The listing builds one solid part. Answer for the finished solid, in the listing's coordinates (mm). Face numbers are marked on the shaded views. A direction names the side the tool comes from. Coordinates: 2 decimals unless noted, no trailing zeros. Write each loop counter-clockwise with the first axis right and the second up, starting at its lowest first coordinate (ties: lowest second). Pieces come first, ordered by that corner, then holes. Notation, with made-up numbers: M -33.5,-2.75 L 18.5,-2.75 A24 cw 18.5,13.25 Z; hole C 34.25,53 d3. An arc over 180 degrees is marked long. Answer as a JSON object with one key per item and string values. Group by question number.
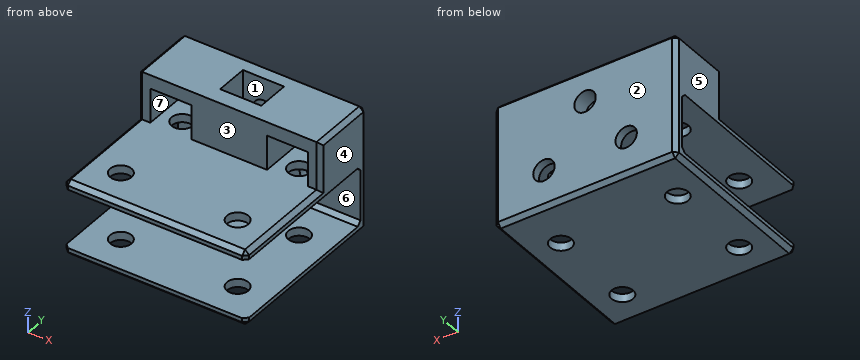
from build123d import *

# Parameters (mm, degrees)
SKETCH1_W           = 44.4
SKETCH1_H           = 40
SKETCH1_R           = 2.6
BOSS_EXTRUDE1_DEPTH = 2
SKETCH2_W           = 44.4
SKETCH2_H           = 18.3
BOSS_EXTRUDE2_DEPTH = 2
LPATTERN1_COUNT     = 2
LPATTERN1_PITCH     = 16.3
SKETCH3_R           = 2.6
CUT_EXTRUDE1_DEPTH  = 64.253853638
BOSS_EXTRUDE3_START = -22.2
SKETCH6_W           = 11.69
SKETCH6_H           = 16
BOSS_EXTRUDE3_DEPTH = 44.4
FILLET4_SIZE        = 1
SKETCH12_W          = 10
SKETCH12_H          = 8.384441544
CUT_EXTRUDE7_DEPTH  = 11
SKETCH11_R          = 2.6
CUT_EXTRUDE8_DEPTH  = 10
CUT_EXTRUDE9_REACH  = 70.079
SKETCH13_W          = 10
SKETCH13_H          = 8


with BuildPart() as part:
    # Sketch1 → Boss-Extrude1 (new body)
    with BuildSketch(Plane.XY):
        with Locations((22.2, 20)):
            Rectangle(SKETCH1_W, SKETCH1_H)
        with Locations((8, 8.476902454)):
            Circle(SKETCH1_R, mode=Mode.SUBTRACT)
        with Locations((8, 29.976902454)):
            Circle(SKETCH1_R, mode=Mode.SUBTRACT)
        with Locations((36.4, 29.976902454)):
            Circle(SKETCH1_R, mode=Mode.SUBTRACT)
        with Locations((36.4, 8.476902454)):
            Circle(SKETCH1_R, mode=Mode.SUBTRACT)
    boss_extrude1 = extrude(amount=BOSS_EXTRUDE1_DEPTH)

    # Sketch2 → Boss-Extrude2 (add)
    with BuildSketch(Plane(origin=(0, 40, 0), x_dir=(1, 0, 0), z_dir=(0, 1, 0))):
        with Locations((22.2, 7.15)):
            Rectangle(SKETCH2_W, SKETCH2_H)
    extrude(amount=BOSS_EXTRUDE2_DEPTH)

    # LPattern1: Boss-Extrude1 ×2
    with Locations(*[(0, 0, -i * LPATTERN1_PITCH) for i in range(1, LPATTERN1_COUNT)]):
        add(boss_extrude1)

    # Sketch3 → Cut-Extrude1 (cut, through all)
    with BuildSketch(Plane(origin=(0, 42, 0), x_dir=(1, 0, 0), z_dir=(0, 1, 0))):
        with Locations(Location((12.2, 7.15, 0), (0, 0, 270))):
            Circle(SKETCH3_R)
        with Locations(Location((32.2, 7.15, 0), (0, 0, 270))):
            Circle(SKETCH3_R)
    extrude(amount=-CUT_EXTRUDE1_DEPTH, mode=Mode.SUBTRACT)

    # Sketch6 → Boss-Extrude3 (add)
    with BuildSketch(Plane(origin=(22.2, 0, 0), x_dir=(0, 0, -1), z_dir=(1, 0, 0)).offset(BOSS_EXTRUDE3_START)):
        with Locations((-7.845, 34)):
            Rectangle(SKETCH6_W, SKETCH6_H)
    extrude(amount=BOSS_EXTRUDE3_DEPTH)

    # Fillet4
    fillet4_edges = [part.edges().sort_by_distance(p)[0] for p in [
        (44.4, 13, 2),
        (0, 21, -16.3),
        (44.4, 21, -16.3),
        (0, 42, -1.305),
        (44.4, 42, -1.305),
        (22.2, 42, -16.3),
        (22.2, 40, -14.3),
        (22.2, 0, -16.3),
        (0, 0, -15.3),
        (44.4, 0, -15.3),
        (22.2, 40, 0),
        (0, 13, 2),
        (44.4, 26, 7.845),
        (44.4, 34, 13.69),
        (22.2, 42, 13.69),
        (0, 26, 7.845),
        (0, 34, 13.69),
        (44.4, 0, 1),
        (0, 0, 1),
        (22.2, 0, 2),
    ]]
    chamfer(fillet4_edges, length=FILLET4_SIZE)

    # Sketch12 → Cut-Extrude7 (cut)
    with BuildSketch(Plane.XZ.offset(-26)):
        with Locations((8, 6.192220772)):
            Rectangle(SKETCH12_W, SKETCH12_H)
        with Locations((36.4, 6.192220772)):
            Rectangle(SKETCH12_W, SKETCH12_H)
    extrude(amount=-CUT_EXTRUDE7_DEPTH, mode=Mode.SUBTRACT)

    # Sketch11 → Cut-Extrude8 (cut)
    with BuildSketch(Plane(origin=(0, 42, 0), x_dir=(1, 0, 0), z_dir=(0, 1, 0))):
        with Locations(Location((22.2, -5.69, 0), (0, 0, 270))):
            Circle(SKETCH11_R)
    extrude(amount=-CUT_EXTRUDE8_DEPTH, mode=Mode.SUBTRACT)

    # Cut-Extrude9: up to this face of the body (flat: up to its plane)
    cut_extrude9_end = Plane(part.part.faces().sort_by_distance((22.2, 16.406575792, 2))[0])
    # Sketch13 → Cut-Extrude9 (cut, up to the picked face)
    with BuildSketch(Plane.XY.offset(13.69), mode=Mode.PRIVATE) as cut_extrude9_sk1:
        with Locations((22.2, 34)):
            Rectangle(SKETCH13_W, SKETCH13_H)
    cut_extrude9_tool1 = split(extrude(cut_extrude9_sk1.sketch, amount=-CUT_EXTRUDE9_REACH, mode=Mode.PRIVATE), bisect_by=cut_extrude9_end, keep=Keep.BOTH, mode=Mode.PRIVATE)
    add(cut_extrude9_tool1.solids().sort_by(Axis((22.2, 34, 13.69), (0, 0, -1)))[0], mode=Mode.SUBTRACT)


solid = part.part
Item 1: For a pull along Y with two mould halves and no side action, classify the marked faces 1, 2, 3 and 4 as +Y half, -Y half, draft (parallel to the pull), parting line (faces both ways), or undercut.
Item 2: A cutting plane is placed at B-B, the plane x = 32.2. Write down the section's boundary in (y, z).
Item 3: A tool of negligible diameter and unlimited length cuts with its end or side. For the marked faces 5, 6 and 7, from which of +Z, -Z, +X, -X, +Y, -Y can it reach the whole face along a straight path? Write none if from no direction.
Item 4: A cutting plane is placed at A-A, the plane z = -7.15. Write down the section's boundary in (x, y).
Item 5: Consider L1, parallel to Y at x = 36.4, z = 0.7; L2, parallel to Z at x = 18.5, y = 17.5; L3, parallel to X at y = 27.5, z = 7. Determine where each line is inside the solid, lowest interval first. Write a range as from..to.
Item 6: A cutting plane is placed at D-D, the plane x = 25.5. Write down the section's boundary in (y, z).
Item 7: A cutting plane is placed at C-C, the plane x = 8. State how many separate pieces and enclosed holes the cut face has, and give its area (3 significant figures).
Item 8: Flat-ended cylindrical pins translate along their axes: pin 1 Ø18 at (x, y) = (13.5, 13.5) entering from +Z; pin 2 Ø11 at (x, z) = (21.5, 9.5) entering from -Y; pin 3 Ø3 at (x, y) = (36.4, 8.48) entering from +Z; pin 4 Ø2.5 at (x, z) = (34, 8) entering from -Y. Find the tip coordinate at first contact, or state that the pin passes through.
Answer:
{
 "1": {"face 1": "undercut", "face 2": "+Y half", "face 3": "-Y half", "face 4": "draft"},
 "2": {"outline": "M 0,-15.3 L 1,-16.3 L 41,-16.3 L 42,-15.3 L 42,-9.75 L 40,-9.75 L 40,-13.3 L 39,-14.3 L 0,-14.3 Z; M 0,0 L 39,0 L 40,-1 L 40,-4.55 L 42,-4.55 L 42,12.69 L 41,13.69 L 26,13.69 L 26,10.38 L 37,10.38 L 37,2 L 1,2 L 0,1 Z"},
 "3": {"face 5": "+Z, -Z, -X, +Y, -Y", "face 6": "+X, -X, -Y", "face 7": "-Y"},
 "4": {"outline": "M 0,40 L 9.6,40 L 9.6,42 L 1,42 L 0,41 Z; M 14.8,40 L 29.6,40 L 29.6,42 L 14.8,42 Z; M 34.8,40 L 44.4,40 L 44.4,41 L 43.4,42 L 34.8,42 Z"},
 "5": {"L1": "0..5.88, 11.08..27.38, 32.58..42", "L2": "-16.3..-14.3, 0..2", "L3": "0..3, 13..31.4, 41.4..44.4"},
 "6": {"outline": "M 0,-15.3 L 1,-16.3 L 41,-16.3 L 42,-15.3 L 42,12.69 L 41,13.69 L 38,13.69 L 38,2 L 30,2 L 30,13.69 L 26,13.69 L 26,2 L 1,2 L 0,1 L 0,0 L 39,0 L 40,-1 L 40,-13.3 L 39,-14.3 L 0,-14.3 Z"},
 "7": {"separate pieces": "5", "enclosed holes": "0", "area": "249 mm2"},
 "8": {"pin 1": "z = 2", "pin 2": "y = 26", "pin 3": "through", "pin 4": "y = 37"}
}
